```python
from build123d import *

# Parameters (mm, degrees)
ESQUISSE1_W        = 5
ESQUISSE1_H        = 3
BOSS_EXTRU_1_DEPTH = 3


with BuildPart() as part:
    # Esquisse1 → Boss.-Extru.1 (new body)
    with BuildSketch(Plane.XY):
        Polygon((-40.414818772, 48.638632865), (-40.414818772, 38.638632865), (-45.414818772, 38.638632865), (-45.414818772, 48.638632865), (-50.414818772, 48.638632865), (-50.414818772, 21.138632865), (-24.414818772, 21.138632865), (-24.414818772, 26.138632865), (-25.414818772, 26.138632865), (-25.414818772, 29.138632865), (-24.414818772, 29.138632865), (-24.414818772, 30.638632865), (-25.414818772, 30.638632865), (-25.414818772, 33.638632865), (-24.414818772, 33.638632865), (-24.414818772, 38.638632865), (-25.414818772, 38.638632865), (-25.414818772, 48.638632865), (-30.414818772, 48.638632865), (-30.414818772, 38.638632865), (-35.414818772, 38.638632865), (-35.414818772, 48.638632865), align=None)
        with Locations((-32.914818772, 27.638632865)):
            Rectangle(ESQUISSE1_W, ESQUISSE1_H, mode=Mode.SUBTRACT)
        with Locations((-42.914818772, 27.638632865)):
            Rectangle(ESQUISSE1_W, ESQUISSE1_H, mode=Mode.SUBTRACT)
        with Locations((-32.914818772, 32.138632865)):
            Rectangle(ESQUISSE1_W, ESQUISSE1_H, mode=Mode.SUBTRACT)
        with Locations((-42.914818772, 32.138632865)):
            Rectangle(ESQUISSE1_W, ESQUISSE1_H, mode=Mode.SUBTRACT)
    extrude(amount=BOSS_EXTRU_1_DEPTH)


solid = part.part
```
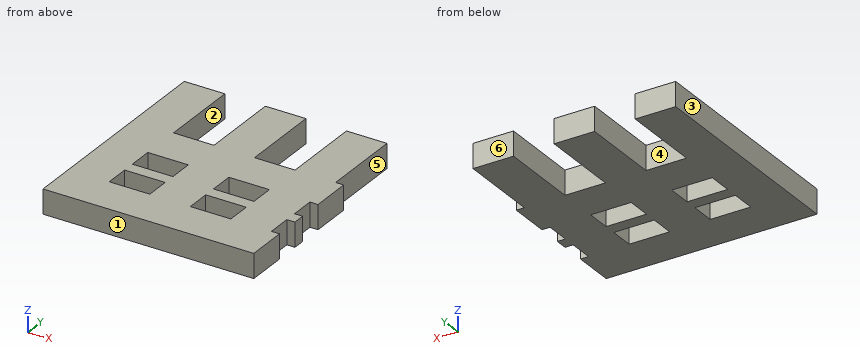
Work out the finished part from the listing and answer in its coordinate system (mm). Face numbers are marked on the shaded views. A direction names the side the tool comes from. Round coordinates to 2 decimals unless told otherwise and drop trailing zeros. Write each loop counter-clockwise with the first axis right and the second up, starting at its lowest first coordinate (ties: lowest second). Pieces come first, ordered by that corner, then holes.
1) A cutting plane is placed at A-A on x = -44.5. Determine the outline of the cut face in (y, z), and give its area (3 significant figures).
2) Consider probe 1 along X at (y, z) = (42.5, 1); probe 2 along Y at (x, z) = (-43.5, 2.2). Determine where each line is inside the solid, lowest interval first.
3) A cutting plane is placed at B-B on y = 43.25. Determine the outline of the cut face in (x, z), and give its area (3 significant figures).
4) Which of the six approach directions +Z, -Z, +X, -X, +Y, -Y give full straight-line access (tool end or side, diameter ignored) to the marked faces 4, 5 and 6?
5) A cutting plane is placed at C-C on z = 2.5. Give the number of separate pieces and of enclosed holes in the cut face, and give its area (3 significant figures).
6) Determine the mould class of the marked faces 1, 2 and 3 for opening direction X: pulls with the +X half, pulls with the -X half, needs draft (parallel to the pull), parting line crosses it, or undercut.
7) Flat-ended cylindrical pins translate along their axes: P1, Ø1.5, axis at y = 28, z = 2, coming from the +X side; P2, Ø0.9, axis at x = -33.5, z = 1, coming from the +Y side. Find the tip coordinate at first contact, or state that the pin passes through.
Entries:
1. outline: (21.14, 0) - (26.14, 0) - (26.14, 3) - (21.14, 3) - close; (29.14, 0) - (30.64, 0) - (30.64, 3) - (29.14, 3) - close; (33.64, 0) - (38.64, 0) - (38.64, 3) - (33.64, 3) - close
1. area: 34.5 mm2
2. probe 1: x = -50.41 to -45.41, -40.41 to -35.41, -30.41 to -25.41
2. probe 2: y = 21.14 to 26.14, 29.14 to 30.64, 33.64 to 38.64
3. outline: (-50.41, 0) - (-45.41, 0) - (-45.41, 3) - (-50.41, 3) - close; (-40.41, 0) - (-35.41, 0) - (-35.41, 3) - (-40.41, 3) - close; (-30.41, 0) - (-25.41, 0) - (-25.41, 3) - (-30.41, 3) - close
3. area: 45.0 mm2
4. face 4: +Z, -Z, +Y
4. face 5: +Z, -Z, +X, +Y
4. face 6: +Z, -Z, +X, -X, +Y
5. separate pieces: 1
5. enclosed holes: 4
5. area: 539 mm2
6. face 1: needs draft
6. face 2: undercut
6. face 3: pulls with the -X half
7. P1: stops at x = -25.41
7. P2: stops at y = 38.64
